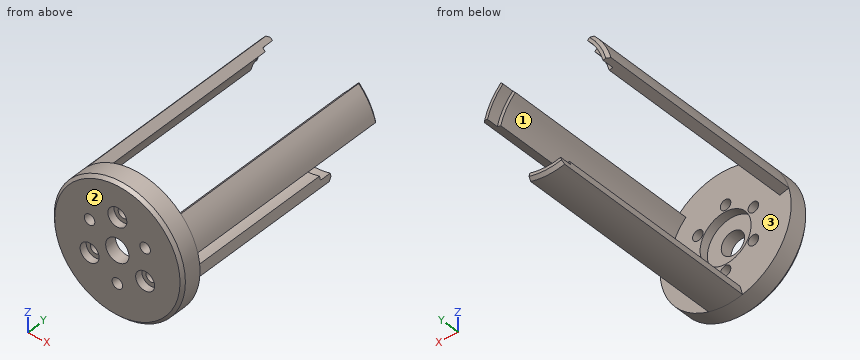
```python
from build123d import *

# Parameters (mm, degrees)
SKETCH1_R           = 22.5
SKETCH1_R_2         = 1.8
SKETCH1_R_3         = 4
BOSS_EXTRUDE1_DEPTH = 7
SKETCH4_R           = 8.75
CUT_EXTRUDE2_DEPTH  = 3
SKETCH6_R           = 3.25
CUT_EXTRUDE3_DEPTH  = 2.5
BOSS_EXTRUDE2_DEPTH = 74
SKETCH7_R           = 20.5
CUT_EXTRUDE4_DEPTH  = 4
CHAMFER2_SIZE       = 1


with BuildPart() as part:
    # Sketch1 → Boss-Extrude1 (new body)
    with BuildSketch(Plane(origin=(0, 0, 0), x_dir=(1, 0, 0), z_dir=(0, 1, 0))):
        Circle(SKETCH1_R)
        with Locations((0, 11)):
            Circle(SKETCH1_R_2, mode=Mode.SUBTRACT)
        with Locations((9.526279442, 5.5)):
            Circle(SKETCH1_R_2, mode=Mode.SUBTRACT)
        with Locations((9.526279442, -5.5)):
            Circle(SKETCH1_R_2, mode=Mode.SUBTRACT)
        with Locations((0, -11)):
            Circle(SKETCH1_R_2, mode=Mode.SUBTRACT)
        with Locations((-9.526279442, -5.5)):
            Circle(SKETCH1_R_2, mode=Mode.SUBTRACT)
        with Locations((-9.526279442, 5.5)):
            Circle(SKETCH1_R_2, mode=Mode.SUBTRACT)
        Circle(SKETCH1_R_3, mode=Mode.SUBTRACT)
    extrude(amount=BOSS_EXTRUDE1_DEPTH)

    # Sketch4 → Cut-Extrude2 (cut)
    with BuildSketch(Plane(origin=(0, 7, 0), x_dir=(1, 0, 0), z_dir=(0, 1, 0))):
        Circle(SKETCH4_R)
    extrude(amount=-CUT_EXTRUDE2_DEPTH, mode=Mode.SUBTRACT)

    # Sketch6 → Cut-Extrude3 (cut)
    with BuildSketch(Plane.XZ):
        with Locations((0, 11)):
            Circle(SKETCH6_R)
        with Locations((9.526279442, -5.5)):
            Circle(SKETCH6_R)
        with Locations((-9.526279442, -5.5)):
            Circle(SKETCH6_R)
    extrude(amount=-CUT_EXTRUDE3_DEPTH, mode=Mode.SUBTRACT)

    # Sketch2 → Boss-Extrude2 (add)
    with BuildSketch(Plane(origin=(0, 7, 0), x_dir=(1, 0, 0), z_dir=(0, 1, 0))):
        with BuildLine():
            Line((4.982266618, 18.594072156), (5.823428515, 21.733331092))
            ThreePointArc((5.823428515, 21.733331092), (0, 22.5), (-5.823428515, 21.733331092))
            Line((-5.823428515, 21.733331092), (-4.982266618, 18.594072156))
            ThreePointArc((-4.982266618, 18.594072156), (0, 19.25), (4.982266618, 18.594072156))
        make_face()
        with BuildLine():
            Line((18.594072156, -4.982266618), (21.733331092, -5.823428515))
            ThreePointArc((21.733331092, -5.823428515), (19.485571585, -11.25), (15.909902577, -15.909902577))
            Line((15.909902577, -15.909902577), (13.611805538, -13.611805538))
            ThreePointArc((13.611805538, -13.611805538), (16.670989023, -9.625), (18.594072156, -4.982266618))
        make_face()
        with BuildLine():
            Line((-13.611805538, -13.611805538), (-15.909902577, -15.909902577))
            ThreePointArc((-15.909902577, -15.909902577), (-19.485571585, -11.25), (-21.733331092, -5.823428515))
            Line((-21.733331092, -5.823428515), (-18.594072156, -4.982266618))
            ThreePointArc((-18.594072156, -4.982266618), (-16.670989023, -9.625), (-13.611805538, -13.611805538))
        make_face()
    extrude(amount=BOSS_EXTRUDE2_DEPTH)

    # Sketch7 → Cut-Extrude4 (cut)
    with BuildSketch(Plane(origin=(0, 81, 0), x_dir=(1, 0, 0), z_dir=(0, 1, 0))):
        Circle(SKETCH7_R)
    extrude(amount=-CUT_EXTRUDE4_DEPTH, mode=Mode.SUBTRACT)

    # Chamfer2
    chamfer2_edges = [part.edges().sort_by_distance(p)[0] for p in [
        (-22.5, 0, 0),
        (19.485571585, 81, 11.25),
        (0, 81, -22.5),
        (-19.485571585, 81, 11.25),
    ]]
    chamfer(chamfer2_edges, length=CHAMFER2_SIZE)


solid = part.part
```
Model file for the job. Use its own axes, mm. Face numbers are marked on the shaded views. A direction names the side the tool comes from. Coordinates: 2 decimals unless noted, no trailing zeros. Order: outer loops, then holes, each group sorted by start corner. A loop starts at its lowest first (then second) coordinate and runs counter-clockwise, first axis right, second up. Notation, with made-up numbers: (68.25, 59.25) -> (120.25, 59.25) arc R21 ccw to (120.25, 81.25) -> close; hole circle Ø7 at (37, 5.5). An arc over 180 degrees is marked (long way). Return JSON: item names as keys, results as strings.
Item 1: Slice it at A-A (z = 0). Write the cut outline in (x, y).
Model answer:
{"outline": "(-22.5, 1) -> (-21.5, 0) -> (-4, 0) -> (-4, 4) -> (-8.75, 4) -> (-8.75, 7) -> (-22.5, 7) -> close; (4, 0) -> (21.5, 0) -> (22.5, 1) -> (22.5, 7) -> (8.75, 7) -> (8.75, 4) -> (4, 4) -> close"}
Item 2: Slice it at B-B (y = 57). Write the cut outline in (x, z).
Model answer:
{"outline": "(-21.73, 5.82) -> (-18.59, 4.98) arc R19.25 cw to (-13.61, 13.61) -> (-15.91, 15.91) arc R22.5 ccw to start; (-5.82, -21.73) arc R22.5 ccw to (5.82, -21.73) -> (4.98, -18.59) arc R19.25 cw to (-4.98, -18.59) -> close; (13.61, 13.61) arc R19.25 cw to (18.59, 4.98) -> (21.73, 5.82) arc R22.5 ccw to (15.91, 15.91) -> close"}
Item 3: Slice it at C-C (z = -5.5). Count the separate pieces of the cut face and the enclosed holes in it, then the cut area to 3 significant figures.
Model answer:
{"separate pieces": "3", "enclosed holes": "0", "area": "199 mm²"}
Item 4: Wall check: line 1 along Z through (x, y) = (0, 4.8); line 2 along Z through (x, y) = (8, 4.5); line 3 along X through (y, z) = (4.9, -5.5). Give the ranges that are in metal, low to high. Write a range as from..to.
Model answer:
{"line 1": "z = -22.5..-12.8, -9.2..-8.75, 8.75..9.2, 12.8..22.5", "line 2": "z = -21.03..-6.45, -4.55..-3.54, 3.54..4.55, 6.45..21.03", "line 3": "x = -21.82..-11.33, -7.73..-6.81, 6.81..7.73, 11.33..21.82"}
Item 5: Pin check, flat tips, straight feed: P1, Ø6, axis at y = 48, z = 12.5, coming from the +X side; P2, Ø10.5, axis at x = -9.53, z = -5.5, coming from the -Y side; P3, Ø1.9, axis at x = -16, z = 8.5, coming from the +Y side; P4, Ø2, axis at y = 68, z = 12, coming from the -X side. Stop position of each tip, or through.
Model answer:
{"P1": "stops at x = 20.4", "P2": "stops at y = 0", "P3": "stops at y = 7", "P4": "stops at x = -19.63"}
Item 6: 3-axis set-ups, long thin cutter, end or side, ignore diameter. For the marked faces 1, 2 and 3: which of +Z, -Z, +X, -X, +Y, -Y reach the whole face in a straight line?
Model answer:
{"face 1": "-Z, +Y", "face 2": "+Z, -Z, +X, -X, -Y", "face 3": "+Y"}
